from build123d import *

# Parameters (mm, degrees)
SKETCH_1_R      = 7
SKETCH_1_R_2    = 4
EXTRUDE_1_DEPTH = 2
SKETCH_2_R      = 7.8
SKETCH_2_R_2    = 4
EXTRUDE_2_DEPTH = 0.8
CHAMFER_1_SIZE  = 0.2


with BuildPart() as part:
    # 草图1 → 凸台-拉伸1 (new body, symmetric)
    with BuildSketch(Plane.XY):
        Circle(SKETCH_1_R)
        Circle(SKETCH_1_R_2, mode=Mode.SUBTRACT)
    extrude(amount=EXTRUDE_1_DEPTH, both=True)

    # 草图2 → 凸台-拉伸2 (add)
    with BuildSketch(Plane.XY.offset(2)):
        Circle(SKETCH_2_R)
        Circle(SKETCH_2_R_2, mode=Mode.SUBTRACT)
    extrude(amount=-EXTRUDE_2_DEPTH)

    # 倒角1
    chamfer_1_edges = [part.edges().sort_by_distance(p)[0] for p in [
        (-7.8, 0, 2),
        (-7.8, 0, 1.2),
        (-7, 0, -2),
    ]]
    chamfer(chamfer_1_edges, length=CHAMFER_1_SIZE)


solid = part.part
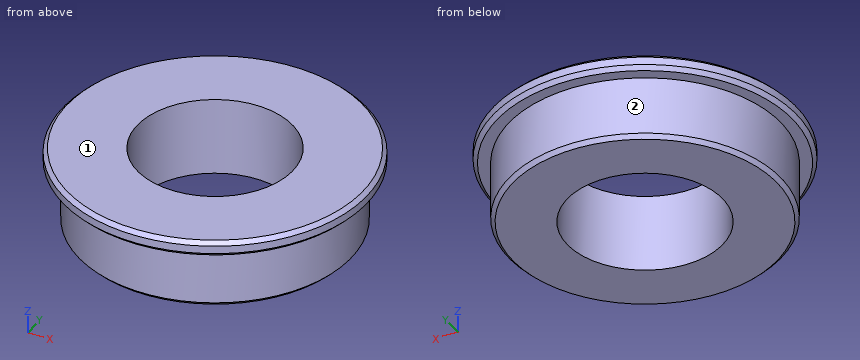
The model under review builds one solid part; all positions refer to its coordinate system, in mm. Face numbers are marked on the shaded views. A direction names the side the tool comes from. Give positions to 0.01 mm unless a question says otherwise; leave off trailing zeros. Loops run counter-clockwise (first coordinate to the right, second up) from the corner with the lowest first, then second, coordinate; pieces in that order, holes last. Notation, with made-up numbers: (27.25, -29) -> (31.25, -29) arc R15 ccw to (31.25, -21) -> close; hole circle Ø5 at (71.5, 65). An arc over 180 degrees is marked (long way). Put each result on its own line as item: value. Start each with the question number.
1. We need section A-A on y = 0. State the section outline as (x, z) points, then the cut area to 3 significant figures.
2. For the marked faces 1 and 2, list the 3-axis set-ups (+Z, -Z, +X, -X, +Y, -Y) from which the entire face can be reached by the end or side of a thin tool; tool diameter is ignored.
3. Clearance check with flat-ended pins moving along their axes: P1, Ø1.5, axis at y = 1.5, z = 0, coming from the +X side; P2, Ø6.5, axis at x = 0, y = 0, coming from the +Z side; P3, Ø2, axis at y = -2, z = 1.5, coming from the +X side. State where each tip first meets the part, or that it passes through.
4. We need section C-C on z = 0.05. State the section outline as (x, y) points.
5. Wall thickness on probe 1 along Y at (x, z) = (0, -0.1); probe 2 along Z at (x, y) = (-4.5, 5.75); probe 3 along Y at (x, z) = (-2, 1.1): over which ranges is each line inside the solid? List them lowest first.
Determined:
1. outline: (-7.8, 1.4) -> (-7.6, 1.2) -> (-7, 1.2) -> (-7, -1.8) -> (-6.8, -2) -> (-4, -2) -> (-4, 2) -> (-7.6, 2) -> (-7.8, 1.8) -> close; (4, -2) -> (6.8, -2) -> (7, -1.8) -> (7, 1.2) -> (7.6, 1.2) -> (7.8, 1.4) -> (7.8, 1.8) -> (7.6, 2) -> (4, 2) -> close
1. area: 25.2 mm^2
2. face 1: +Z, +X, -X, +Y, -Y
2. face 2: -Z
3. P1: x = 6.96
3. P2: through
3. P3: x = 7.74
4. outline: circle Ø14 at (0, 0); hole circle Ø8 at (0, 0)
5. probe 1: -7 to -4, 4 to 7
5. probe 2: 1.2 to 2
5. probe 3: -6.71 to -3.46, 3.46 to 6.71
